Work out the finished part from the listing and answer in its coordinate system (mm). A direction names the side the tool comes from. Coordinates: 2 decimals unless noted, no trailing zeros. Loops run counter-clockwise (first coordinate to the right, second up) from the corner with the lowest first, then second, coordinate; pieces in that order, holes last.
```python
from build123d import *

# Parameters (mm, degrees)
F1_DEPTH = 13
F2_SIZE  = 0.2


with BuildPart() as f1:
    # F0 (on Top) → F1 (new body)
    with BuildSketch(Plane.XY):
        with BuildLine():
            ThreePointArc((-1.8816, -16.819208), (-0.9408, -17.760008), (0, -16.819208))
            Line((0, -16.819208), (0, 0))
            Line((0, 0), (5, 0))
            Line((5, 0), (5, -7))
            ThreePointArc((5, -7), (1.440063, -11.456932), (1.566748, -17.159682))
            ThreePointArc((1.566748, -17.159682), (2.784253, -17.696238), (3.320809, -16.478734))
            ThreePointArc((3.320809, -16.478734), (3.298597, -11.846796), (6.374464, -8.383506))
            ThreePointArc((6.374464, -8.383506), (6.744882, -8.037039), (6.8816, -7.548616))
            Line((6.8816, -7.548616), (6.8816, 0.9408))
            ThreePointArc((6.8816, 0.9408), (6.606046, 1.606046), (5.9408, 1.8816))
            Line((5.9408, 1.8816), (-0.779544, 1.8816))
            ThreePointArc((-0.779544, 1.8816), (-1.546355, 1.674728), (-1.8816, 0.954723))
            Line((-1.8816, 0.954723), (-1.8816, -0.573602))
            ThreePointArc((-1.8816, -0.573602), (-2.508632, -3.043383), (-4.237854, -4.914955))
            ThreePointArc((-4.237854, -4.914955), (-4.464092, -5.866265), (-3.524931, -6.13857))
            ThreePointArc((-3.524931, -6.13857), (-1.8816, -7.137048), (-3.524931, -8.135526))
            ThreePointArc((-3.524931, -8.135526), (-4.464092, -8.407832), (-4.237854, -9.359142))
            ThreePointArc((-4.237854, -9.359142), (-2.508632, -11.230713), (-1.8816, -13.700494))
            Line((-1.8816, -13.700494), (-1.8816, -16.819208))
        make_face()
    extrude(amount=F1_DEPTH)

    # F2
    f2_edges = [f1.edges().sort_by_distance(p)[0] for p in [
        (-2.508632, -11.230713, 0),
        (-1.8816, -15.259851, 0),
        (-0.9408, -17.760008, 0),
        (0, -8.409604, 0),
        (2.5, 0, 0),
        (5, -3.5, 0),
        (1.440063, -11.456932, 0),
        (2.784253, -17.696238, 0),
        (3.298597, -11.846796, 0),
        (6.744882, -8.037039, 0),
        (6.8816, -3.303908, 0),
        (6.606046, 1.606046, 0),
        (2.580628, 1.8816, 0),
        (-1.546355, 1.674728, 0),
        (-1.8816, 0.19056, 0),
        (-2.508632, -3.043383, 0),
        (-4.464092, -5.866265, 0),
        (-1.8816, -7.137048, 0),
        (-4.464092, -8.407832, 0),
        (-2.508632, -11.230713, 13),
        (-1.8816, -15.259851, 13),
        (-0.9408, -17.760008, 13),
        (0, -8.409604, 13),
        (2.5, 0, 13),
        (5, -3.5, 13),
        (1.440063, -11.456932, 13),
        (2.784253, -17.696238, 13),
        (3.298597, -11.846796, 13),
        (6.744882, -8.037039, 13),
        (6.8816, -3.303908, 13),
        (6.606046, 1.606046, 13),
        (2.580628, 1.8816, 13),
        (-1.546355, 1.674728, 13),
        (-1.8816, 0.19056, 13),
        (-2.508632, -3.043383, 13),
        (-4.464092, -5.866265, 13),
        (-1.8816, -7.137048, 13),
        (-4.464092, -8.407832, 13),
    ]]
    chamfer(f2_edges, length=F2_SIZE)


solid = f1.part
```
1. Straight lines are drawn through the part: probe 1 along X at (y, z) = (-0.25, 9.75); probe 2 along X at (y, z) = (0.5, 4.5); probe 3 along X at (y, z) = (-7.25, 5.25). For each, find the intervals that lie inside material, in ascending order.
2. For faces 1 (the flat face through (-1.882, -15, 6)), 2 (the cylindrical face through (6.61, 1.6, 6.41)), 3 (the cylindrical face through (1.467, -11.38, 6.412)), 4 (the flat face through (0, -9, 6)), determine the directions among +Z, -Z, +X, -X, +Y, -Y from which every point of the face is accessible in a straight line to the end or side of a thin tool.
3. Determine the mould class of faces 5 (the flat face through (2, 0, 6)), 6 (the flat face through (6.882, -3, 6)), 7 (the flat face through (-1, -6, 13)) for opening direction X: released by +X, released by -X, zero draft, split by the parting line, or undercut.
4. A cutting plane is placed at A-A, the plane x = 0.25. Give the vertices of the cut face in (y, z), then the cut area to 3 significant figures.
5. Each of these flat-tipped pins is pushed along its axis until it touches: P1, Ø1.4, axis at x = -3.01, y = -7.14, coming from the -Z side; P2, Ø1, axis at y = -11.5, z = 11, coming from the -X side; P3, Ø1.5, axis at y = -7.5, z = 4.5, coming from the -X side; P4, Ø3.5, axis at x = 2, z = 7, coming from the +Y side. Where does it stop, or does it pass through?
Answers below:
1. probe 1: x = -1.88 to 0, 5 to 6.88
1. probe 2: x = -1.88 to 6.88
1. probe 3: x = -1.89 to 0, 4.62 to 6.88
2. face 1: +Z, -Z, -X, -Y
2. face 2: +Z, -Z, +X, +Y
2. face 3: +Z, -Z
2. face 4: +Z, -Z, -Y
3. face 5: undercut
3. face 6: released by +X
3. face 7: zero draft
4. outline: (0, 0.2) - (0.2, 0) - (1.68, 0) - (1.88, 0.2) - (1.88, 12.8) - (1.68, 13) - (0.2, 13) - (0, 12.8) - close
4. area: 24.4 mm2
5. P1: passes through
5. P2: stops at x = -2.64
5. P3: stops at x = -4.34
5. P4: stops at y = 1.88
